Read the model definition and answer for the solid it produces. Units are mm, in the model's axes. Round coordinates to 2 decimals unless told otherwise and drop trailing zeros. Write each loop counter-clockwise with the first axis right and the second up, starting at its lowest first coordinate (ties: lowest second). Pieces come first, ordered by that corner, then holes. Notation, with made-up numbers: (82, 63.25) - (122, 63.25) arc R28 ccw to (122, 86.25) - close; hole circle Ø8 at (2.5, 35). An arc over 180 degrees is marked (long way). Use one line per item in the form item = value. Start each with the question number.
1) Each of these flat-tipped pins is pushed along its axis until it touches: pin 1 (6 mm diameter, centred on x = 11, y = -21, fed in from +Z); pin 2 (8 mm diameter, centred on y = 36.5, z = -8.5, fed in from +X); pin 3 (23 mm diameter, centred on y = -6.5, z = -2.5, fed in from -X); pin 4 (6 mm diameter, centred on x = 20, y = 4.5, fed in from +Z). Where does it stop, or does it pass through?
2) Consider line 1 along Z through (x, y) = (27.5, 20); line 2 along Z through (x, y) = (38, -23); line 3 along Y through (x, z) = (34, 32.5). Determine where each line is inside the solid, lowest interval first. Write a range as from..to.
3) The part is cut by section C-C, the plane z = 46. Give the vertices of the cut face in (x, y).
4) The part is cut by section B-B, the plane y = -32. Give the vertices of the cut face in (x, z), plus the area to 3 significant figures.
5) For a pull along Z with two mould halves and no side action, classify faces 1 (the face through (5.4, -3.9, -5.5)), 2 (the face through (5.4, -0.02, 6.74)), 3 (the face through (39.491, -50, -4)) as released by +Z, released by -Z, zero draft, split by the parting line, or undercut.
6) The part is cut by section A-A, the plane x = 22. Give the vertices of the cut face in (y, z), plus the area to 3 significant figures.
from build123d import *

# Parameters (mm, degrees)
F2_T = -6.35
F3_W = 12.7568915486
F3_H = 15.9924589097


# Not quite as in the source:
# - a feature names something its author has since deleted; it is built from what else it names


with BuildPart() as f1:
    # F0 (on Front) → F1 (revolve)
    with BuildSketch(Plane.XZ):
        with BuildLine():
            Line((39.4908925979, 0), (39.4908925979, 56.4475917369))
            ThreePointArc((39.4908925979, 56.4475917369), (14.1063703184, 33.1501751178), (4.71438, 0))
            Line((4.71438, 0), (39.4908925979, 0))
        make_face()
    revolve(axis=Axis((0, 0, 0), (1, 0, 0)))

    # F2
    f2_openings = [f1.faces().sort_by_distance(p)[0] for p in [
        (39.490893, 0, 0),
    ]]
    offset(amount=F2_T, openings=f2_openings)

    # F3 (on Front) → F4 (revolve, cut)
    with BuildSketch(Plane.XZ):
        with Locations((0, 7.9962294549)):
            Rectangle(F3_W, F3_H)
    revolve(axis=Axis((0, 0, 0), (1, 0, 0)), mode=Mode.SUBTRACT)

    # F5 (on face) → F6 (revolve)
    with BuildSketch(Plane(origin=(6.3784457743, 0, 0), x_dir=(0, -1, 0), z_dir=(-1, 0, 0))):
        Polygon((-1.9871168115, 13.66252359), (0, 0), (0, 13.66252359), align=None)
    revolve(axis=Axis((6.3784457743, 0, 6.831261795), (0, 0, -1)))

    # F5 (on face) → F7 (revolve)
    with BuildSketch(Plane(origin=(6.3784457743, 0, 0), x_dir=(0, -1, 0), z_dir=(-1, 0, 0))):
        Polygon((-8.0306298753, 11.0532137704), (0, 0), (-6.423018605, 12.2212117268), align=None)
    revolve(axis=Axis((6.3784457743, 4.0153149377, 5.5266068852), (0, -0.5877852523, -0.8090169944)))

    # F5 (on face) → F8 (revolve)
    with BuildSketch(Plane(origin=(6.3784457743, 0, 0), x_dir=(0, -1, 0), z_dir=(-1, 0, 0))):
        Polygon((-12.9938320893, 4.2219519754), (0, 0), (-12.3797792248, 6.1118123676), align=None)
    revolve(axis=Axis((6.3784457743, 6.4969160447, 2.1109759877), (0, -0.9510565163, -0.3090169944)))

    # F5 (on face) → F9 (revolve)
    with BuildSketch(Plane(origin=(6.3784457743, 0, 0), x_dir=(0, -1, 0), z_dir=(-1, 0, 0))):
        Polygon((-12.9938320893, -4.2219519754), (0, 0), (-13.6078849539, -2.3320915832), align=None)
    revolve(axis=Axis((6.3784457743, 6.4969160447, -2.1109759877), (0, -0.9510565163, 0.3090169944)))

    # F5 (on face) → F10 (revolve)
    with BuildSketch(Plane(origin=(6.3784457743, 0, 0), x_dir=(0, -1, 0), z_dir=(-1, 0, 0))):
        Polygon((-8.0306298753, -11.0532137704), (0, 0), (-9.6382411456, -9.885215814), align=None)
    revolve(axis=Axis((6.3784457743, 4.0153149377, -5.5266068852), (0, -0.5877852523, 0.8090169944)))

    # F5 (on face) → F11 (revolve)
    with BuildSketch(Plane(origin=(6.3784457743, 0, 0), x_dir=(0, -1, 0), z_dir=(-1, 0, 0))):
        Polygon((0, -13.66252359), (0, 0), (-1.9871168115, -13.66252359), align=None)
    revolve(axis=Axis((6.3784457743, 0, -6.831261795), (0, 0, 1)))

    # F5 (on face) → F12 (revolve)
    with BuildSketch(Plane(origin=(6.3784457743, 0, 0), x_dir=(0, -1, 0), z_dir=(-1, 0, 0))):
        Polygon((6.423018605, 12.2212117268), (0, 0), (8.0306298753, 11.0532137704), align=None)
    revolve(axis=Axis((6.3784457743, -4.0153149377, 5.5266068852), (0, 0.5877852523, -0.8090169944)))

    # F5 (on face) → F13 (revolve)
    with BuildSketch(Plane(origin=(6.3784457743, 0, 0), x_dir=(0, -1, 0), z_dir=(-1, 0, 0))):
        Polygon((12.3797792248, 6.1118123676), (0, 0), (12.9938320893, 4.2219519754), align=None)
    revolve(axis=Axis((6.3784457743, -6.4969160447, 2.1109759877), (0, 0.9510565163, -0.3090169944)))

    # F5 (on face) → F14 (revolve)
    with BuildSketch(Plane(origin=(6.3784457743, 0, 0), x_dir=(0, -1, 0), z_dir=(-1, 0, 0))):
        Polygon((13.6078849539, -2.3320915832), (0, 0), (12.9938320893, -4.2219519754), align=None)
    revolve(axis=Axis((6.3784457743, -6.4969160447, -2.1109759877), (0, 0.9510565163, 0.3090169944)))

    # F5 (on face) → F15 (revolve)
    with BuildSketch(Plane(origin=(6.3784457743, 0, 0), x_dir=(0, -1, 0), z_dir=(-1, 0, 0))):
        Polygon((9.6382411456, -9.885215814), (0, 0), (8.0306298753, -11.0532137704), align=None)
    revolve(axis=Axis((6.3784457743, -4.0153149377, -5.5266068852), (0, 0.5877852523, 0.8090169944)))


solid = f1.part
Geometry results:
q1.pin_1 = 25.86
q1.pin_2 = 29.04
q1.pin_3 = 4.39
q1.pin_4 = 44.25
q2.line_1 = -44.28..-34.62, 34.62..44.28
q2.line_2 = -50.7..-42.52, 42.52..50.7
q2.line_3 = -42.28..-32.02, 32.02..42.28
q3.outline = (39.49, -32.72) - (39.49, -17.55) arc R33.41 cw to (39.49, 17.55) - (39.49, 32.72) arc R43.34 ccw to start
q4.outline = (39.49, -46.5) - (39.49, -37.42) arc R46.99 cw to (39.49, 37.42) - (39.49, 46.5) arc R54.5 ccw to start
q4.area = 744 mm2
q5.face_1 = undercut
q5.face_2 = undercut
q5.face_3 = zero draft
q6.outline = circle Ø86.86 at (0, 0); hole circle Ø67.05 at (0, 0)
q6.area = 2,390 mm2
